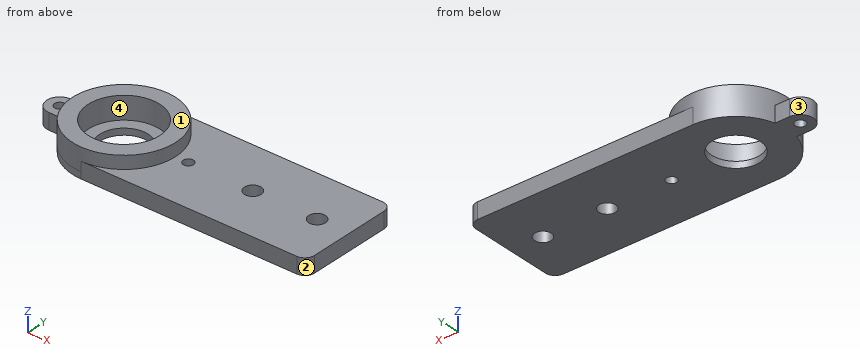
from build123d import *

# Parameters (mm, degrees)
SKETCH3_R           = 7.5
BOSS_EXTRUDE3_DEPTH = 2
SKETCH2_R           = 16
SKETCH2_R_2         = 11.1
BOSS_EXTRUDE4_DEPTH = 9
SKETCH4_R           = 2.6
BOSS_EXTRUDE5_DEPTH = 5
FILLET3_R           = 3
SKETCH5_R           = 1.6
BOSS_EXTRUDE6_DEPTH = 5
SKETCH6_R           = 1.6
CUT_EXTRUDE1_DEPTH  = 10


with BuildPart() as part:
    # Sketch3 → Boss-Extrude3 (new body)
    with BuildSketch(Plane.XY):
        with BuildLine():
            Line((-15.491933385, 4), (-15.491933385, -4))
            ThreePointArc((-15.491933385, -4), (16, 0), (-15.491933385, 4))
        make_face()
        Circle(SKETCH3_R, mode=Mode.SUBTRACT)
    extrude(amount=BOSS_EXTRUDE3_DEPTH)

    # Sketch2 → Boss-Extrude4 (add)
    with BuildSketch(Plane.XY):
        Circle(SKETCH2_R)
        Circle(SKETCH2_R_2, mode=Mode.SUBTRACT)
    extrude(amount=BOSS_EXTRUDE4_DEPTH)

    # Sketch4 → Boss-Extrude5 (add)
    with BuildSketch(Plane.XY):
        with BuildLine():
            Line((70, 16), (30, 16))
            Line((30, 16), (0, 16))
            ThreePointArc((0, 16), (11.313708499, 11.313708499), (16, 0))
            ThreePointArc((16, 0), (11.313708499, -11.313708499), (0, -16))
            Line((0, -16), (70, -16))
            Line((70, -16), (70, 16))
        make_face()
        with Locations((40, 0)):
            Circle(SKETCH4_R, mode=Mode.SUBTRACT)
        with Locations((60, 0)):
            Circle(SKETCH4_R, mode=Mode.SUBTRACT)
    extrude(amount=BOSS_EXTRUDE5_DEPTH)

    # Fillet3
    fillet3_edges = [part.edges().sort_by_distance(p)[0] for p in [
        (70, -16, 2.5),
        (70, 16, 2.5),
    ]]
    fillet(fillet3_edges, radius=FILLET3_R)

    # Sketch5 → Boss-Extrude6 (add)
    with BuildSketch(Plane.XY):
        with BuildLine():
            Line((-20, 4), (-15.491933385, 4))
            Line((-15.491933385, 4), (-15.491933385, -4))
            Line((-15.491933385, -4), (-20, -4))
            ThreePointArc((-20, -4), (-24, 0), (-20, 4))
        make_face()
        with Locations((-20, 0)):
            Circle(SKETCH5_R, mode=Mode.SUBTRACT)
    extrude(amount=BOSS_EXTRUDE6_DEPTH)

    # Sketch6 → Cut-Extrude1 (cut)
    with BuildSketch(Plane.XY.offset(5)):
        with Locations((20, 0)):
            Circle(SKETCH6_R)
    extrude(amount=-CUT_EXTRUDE1_DEPTH, mode=Mode.SUBTRACT)


solid = part.part
CAD build for the part. Positions are in the model's coordinates, mm. Face numbers are marked on the shaded views. Give positions to 0.01 mm unless a question says otherwise; leave off trailing zeros. Write each loop counter-clockwise with the first axis right and the second up, starting at its lowest first coordinate (ties: lowest second). Pieces come first, ordered by that corner, then holes. Notation, with made-up numbers: (31.5, -11) - (35.5, -11) arc R30 cw to (35.5, 22) - close; hole circle Ø9 at (-6.5, -5.5). An arc over 180 degrees is marked (long way). Put each result on its own line as item: value.
(1) Pull direction X, two halves, no side cores. Call the marked faces 1, 2, 3 and 4: released by +X, released by -X, zero draft, split by the parting line, or undercut.
Working result:
face 1: zero draft
face 2: released by +X
face 3: released by -X
face 4: undercut
(2) Drop flat-ended pins along their axis: pin 1 Ø4 at (x, y) = (-19.5, 1) entering from +Z; pin 2 Ø1.4 at (x, z) = (-17, 2) entering from +Y; pin 3 Ø1.5 at (x, z) = (-6, 6.5) entering from -Y; pin 4 Ø3 at (x, y) = (-20, 0) entering from -Z. Give the stop position or say it passes through.
Working result:
pin 1: z = 5
pin 2: y = 4
pin 3: y = -15.11
pin 4: through
(3) Saw through at A-A (x = 20). List the corners of the cut face in (y, z).
Working result:
outline: (-16, 0) - (-1.6, 0) - (-1.6, 5) - (-16, 5) - close; (1.6, 0) - (16, 0) - (16, 5) - (1.6, 5) - close
(4) Saw through at D-D (y = 10). List the corners of the cut face in (x, z), then the cut area to 3 significant figures.
Working result:
outline: (-12.49, 0) - (70, 0) - (70, 5) - (12.49, 5) - (12.49, 9) - (4.82, 9) - (4.82, 2) - (-4.82, 2) - (-4.82, 9) - (-12.49, 9) - close
area: 445 mm^2
(5) Wall check: L1, parallel to Y at x = -20, z = 1.25; L2, parallel to Y at x = 60, z = 2.95; L3, parallel to Z at x = 32, y = 3.5. Give the ranges that are in metal, low to high.
Working result:
L1: -4 to -1.6, 1.6 to 4
L2: -16 to -2.6, 2.6 to 16
L3: 0 to 5
(6) Saw through at B-B (z = 4). List the corners of the cut face in (x, y), then the cut area to 3 significant figures.
Working result:
outline: (-20, -4) - (-15.49, -4) arc R16 ccw to (0, -16) - (67, -16) arc R3 ccw to (70, -13) - (70, 13) arc R3 ccw to (67, 16) - (0, 16) arc R16 ccw to (-15.49, 4) - (-20, 4) arc R4 ccw to start; hole circle Ø3.2 at (-20, 0); hole circle Ø22.2 at (0, 0); hole circle Ø3.2 at (20, 0); hole circle Ø5.2 at (40, 0); hole circle Ø5.2 at (60, 0)
area: 2,250 mm^2
(7) Saw through at C-C (x = 46.5). List the corners of the cut face in (y, z).
Working result:
outline: (-16, 0) - (16, 0) - (16, 5) - (-16, 5) - close
